```python
from build123d import *

# Parameters (mm, degrees)
EXTRUDE_1_DEPTH              = 20
CUT_EXTRUDE_1_REACH          = 50.59
SKETCH_8_W                   = 11
SKETCH_8_H                   = 6
HOLE_WIZARD_M6_3_D           = 5
HOLE_WIZARD_M6_3_DEPTH       = 35
HOLE_WIZARD_M6_3_CSINK_D     = 6.05
HOLE_WIZARD_M6_3_CSINK_ANGLE = 90
HOLE_WIZARD_M6_3_TIP         = 1.502151548
SKETCH_13_R                  = 3
CUT_EXTRUDE_2_DEPTH          = 45
CUT_EXTRUDE_3_DEPTH          = 7
CHAMFER_1_SIZE               = 2
SKETCH_15_R                  = 1.5
CUT_EXTRUDE_4_DEPTH          = 10


with BuildPart() as part:
    # 草图1 → 凸台-拉伸1 (new, symmetric)
    with BuildSketch(Plane.XY):
        Polygon((-10, 5), (10, 5), (7.75, 0), (20, 0), (20, 19), (-20, 19), (-20, 0), (-7.75, 0), align=None)
    extrude(amount=EXTRUDE_1_DEPTH, both=True)

    # 草图8 → 切除-拉伸1 (cut, up to next)
    with BuildSketch(Plane(origin=(0, 0, -20), x_dir=(-1, 0, 0), z_dir=(0, 0, -1)), mode=Mode.PRIVATE) as cut_extrude_1_sk1:
        with Locations((0, 5)):
            Rectangle(SKETCH_8_W, SKETCH_8_H)
    cut_extrude_1_tool1 = extrude(cut_extrude_1_sk1.sketch, amount=-CUT_EXTRUDE_1_REACH, mode=Mode.PRIVATE) & part.part
    add(cut_extrude_1_tool1.solids().sort_by_distance((0, 5, -20))[0], mode=Mode.SUBTRACT)

    # M6 螺纹孔3
    with Locations(Plane.ZY.offset(20)):
        with Locations((0, 6)):
            CounterSinkHole(HOLE_WIZARD_M6_3_D / 2, HOLE_WIZARD_M6_3_CSINK_D / 2, depth=HOLE_WIZARD_M6_3_DEPTH, counter_sink_angle=HOLE_WIZARD_M6_3_CSINK_ANGLE)
            with Locations((0, 0, -(HOLE_WIZARD_M6_3_DEPTH + HOLE_WIZARD_M6_3_TIP / 2))):  # 118° drill point
                Cone(0, HOLE_WIZARD_M6_3_D / 2, HOLE_WIZARD_M6_3_TIP, mode=Mode.SUBTRACT)

    # 草图13 → 切除-拉伸2 (cut)
    with BuildSketch(Plane(origin=(20, 0, 0), x_dir=(0, 0, -1), z_dir=(1, 0, 0))):
        with Locations((0, 9)):
            Circle(SKETCH_13_R)
    extrude(amount=-CUT_EXTRUDE_2_DEPTH, mode=Mode.SUBTRACT)

    # 草图14 → 切除-拉伸3 (cut)
    with BuildSketch(Plane.XZ.offset(-8)):
        with BuildLine():
            Line((5.5, 5.5), (5.5, -5.5))
            ThreePointArc((5.5, -5.5), (0, -11), (-5.5, -5.5))
            Line((-5.5, -5.5), (-5.5, 5.5))
            ThreePointArc((-5.5, 5.5), (0, 11), (5.5, 5.5))
        make_face()
    extrude(amount=-CUT_EXTRUDE_3_DEPTH, mode=Mode.SUBTRACT)

    # 倒角1
    chamfer_1_edges = [part.edges().sort_by_distance(p)[0] for p in [
        (20, 9.5, 20),
        (-20, 9.5, 20),
        (-20, 9.5, -20),
        (20, 9.5, -20),
    ]]
    chamfer(chamfer_1_edges, length=CHAMFER_1_SIZE)

    # 草图15 → 切除-拉伸4 (cut)
    with BuildSketch(Plane(origin=(0, 19, 0), x_dir=(1, 0, 0), z_dir=(0, 1, 0))):
        with Locations(Location((-16, 16, 0), (0, 0, 270))):
            Circle(SKETCH_15_R)
        with Locations(Location((16, 16, 0), (0, 0, 270))):
            Circle(SKETCH_15_R)
        with Locations(Location((16, -16, 0), (0, 0, 270))):
            Circle(SKETCH_15_R)
        with Locations(Location((-16, -16, 0), (0, 0, 270))):
            Circle(SKETCH_15_R)
    extrude(amount=-CUT_EXTRUDE_4_DEPTH, mode=Mode.SUBTRACT)


solid = part.part
```
Here's how the part is built. I have some questions about the finished solid (model axes, mm). A direction names the side the tool comes from. Round coordinates to 2 decimals unless told otherwise and drop trailing zeros. Order: outer loops, then holes, each group sorted by start corner. A loop starts at its lowest first (then second) coordinate and runs counter-clockwise, first axis right, second up. Notation, with made-up numbers: M 63,9 L 101,9 A31 cw 101,42 Z; hole C 68.5,16.25 d3. An arc over 180 degrees is marked long. Answer as CSV lines item,"result".
Item 1: Imagine slicing it at D-D on z = 16. List the corners of the cut face in (x, y) for me.
From the geometry:
outline,"M -20,0 L -7.75,0 L -10,5 L -5.5,5 L -5.5,8 L 5.5,8 L 5.5,5 L 10,5 L 7.75,0 L 20,0 L 20,19 L 17.5,19 L 17.5,9 L 14.5,9 L 14.5,19 L -14.5,19 L -14.5,9 L -17.5,9 L -17.5,19 L -20,19 Z"
Item 2: We'd pull the mould along Z, two halves only. Please class faces 4 (the flat face through (8, 5, 11)), 5 (the flat face through (0, 12, -20)), 6 (the flat face through (5.5, 12.2, -0.3)): +Z half, -Z half, draft (parallel to the pull), parting line (faces both ways), or undercut.
From the geometry:
face 4,"draft"
face 5,"-Z half"
face 6,"undercut"
Item 3: Please list where these lines run through material, in increasing order: L1, parallel to X at y = 16.75, z = 16; L2, parallel to Z at x = -11, y = 8.75; L3, parallel to Y at x = -10.5, z = 0. Write a range as [from, to].
From the geometry:
L1,"[-20, -17.5], [-14.5, 14.5], [17.5, 20]"
L2,"[-20, -2.99], [2.99, 20]"
L3,"[0, 3.5], [12, 19]"
Item 4: Imagine slicing it at A-A on y = 16.5. List the corners of the cut face in (x, z) for me, and give its area (3 significant figures).
From the geometry:
outline,"M -20,-18 L -18,-20 L 18,-20 L 20,-18 L 20,18 L 18,20 L -18,20 L -20,18 Z; hole C -16,-16 d3; hole C -16,16 d3; hole C 16,-16 d3; hole C 16,16 d3"
area,"1,560 mm2"
Item 5: For pin 1 (1.5 mm diameter, centred on x = 4, z = 10.5, fed in from -Y); pin 2 (1.5 mm diameter, centred on x = 16, z = 16.5, fed in from +Y); pin 3 (4 mm diameter, centred on y = 6, z = 0, fed in from -X), each with a flat end and sliding along its axis, tell me the tip position at first contact or that it passes through.
From the geometry:
pin 1,"y = 8"
pin 2,"y = 9"
pin 3,"x = 15.3"
Item 6: Which directions (+Z, -Z, +X, -X, +Y, -Y) give clear straight access to the entire face, cutting with the end or side of a thin tool? Please do faces 1 (the cylindrical face through (16.07, 14.07, -17.5)), 2 (the cylindrical face through (11.4, 3.5, 0.1)), 3 (the flat face through (0, 15, 0)).
From the geometry:
face 1,"+Y"
face 2,"-X"
face 3,"-Y"
Item 7: Imagine slicing it at B-B on y = 13. List the corners of the cut face in (x, z) for me, and give its area (3 significant figures).
From the geometry:
outline,"M -20,-18 L -18,-20 L 18,-20 L 20,-18 L 20,18 L 18,20 L -18,20 L -20,18 Z; hole C -16,-16 d3; hole C -16,16 d3; hole M -5.5,-5.5 A5.5 ccw 5.5,-5.5 L 5.5,5.5 A5.5 ccw -5.5,5.5 Z; hole C 16,-16 d3; hole C 16,16 d3"
area,"1,350 mm2"
Item 8: Imagine slicing it at C-C on x = 16. List the corners of the cut face in (y, z) for me, and give its area (3 significant figures).
From the geometry:
outline,"M 0,-20 L 19,-20 L 19,-17.5 L 9,-17.5 L 9,-14.5 L 19,-14.5 L 19,14.5 L 9,14.5 L 9,17.5 L 19,17.5 L 19,20 L 0,20 Z; hole M 6.12,-0.83 A3 ccw long 6.12,0.83 A0.84 ccw long Z"
area,"671 mm2"
